from build123d import *

# Parameters (mm, degrees)
SKETCH_1_R          = 20
EXTRUDE_1_DEPTH     = 5
SKETCH_2_R          = 2
CUT_EXTRUDE_1_DEPTH = 29.722813233
SKETCH_3_R          = 3.5
CUT_EXTRUDE_2_DEPTH = 3
SKETCH_4_R          = 3
EXTRUDE_2_DEPTH     = 8
CUT_EXTRUDE_START   = -5
CUT_EXTRUDE_3_DEPTH = 5


with BuildPart() as part:
    # 草图1 → 凸台-拉伸1 (new body)
    with BuildSketch(Plane(origin=(0, 0, 0), x_dir=(1, 0, 0), z_dir=(0, 1, 0))):
        with Locations(Location((0, 0, 0), (0, 0, 270))):
            Circle(SKETCH_1_R)
    extrude(amount=EXTRUDE_1_DEPTH)

    # 草图2 → 切除-拉伸1 (cut, through all)
    with BuildSketch(Plane(origin=(0, 5, 0), x_dir=(1, 0, 0), z_dir=(0, 1, 0))):
        with Locations(Location((14, 0, 0), (0, 0, 270))):
            Circle(SKETCH_2_R)
        with Locations(Location((7, -12.124355653, 0), (0, 0, 270))):
            Circle(SKETCH_2_R)
        with Locations(Location((-7, -12.124355653, 0), (0, 0, 270))):
            Circle(SKETCH_2_R)
        with Locations(Location((-14, 0, 0), (0, 0, 270))):
            Circle(SKETCH_2_R)
        with Locations(Location((-7, 12.124355653, 0), (0, 0, 270))):
            Circle(SKETCH_2_R)
        with Locations(Location((7, 12.124355653, 0), (0, 0, 270))):
            Circle(SKETCH_2_R)
    extrude(amount=-CUT_EXTRUDE_1_DEPTH, mode=Mode.SUBTRACT)

    # 草图3 → 切除-拉伸2 (cut)
    with BuildSketch(Plane(origin=(0, 5, 0), x_dir=(1, 0, 0), z_dir=(0, 1, 0))):
        with Locations(Location((14, 0, 0), (0, 0, 270))):
            Circle(SKETCH_3_R)
        with Locations(Location((7, -12.124355653, 0), (0, 0, 270))):
            Circle(SKETCH_3_R)
        with Locations(Location((-7, -12.124355653, 0), (0, 0, 270))):
            Circle(SKETCH_3_R)
        with Locations(Location((-14, 0, 0), (0, 0, 270))):
            Circle(SKETCH_3_R)
        with Locations(Location((-7, 12.124355653, 0), (0, 0, 270))):
            Circle(SKETCH_3_R)
        with Locations(Location((7, 12.124355653, 0), (0, 0, 270))):
            Circle(SKETCH_3_R)
    extrude(amount=-CUT_EXTRUDE_2_DEPTH, mode=Mode.SUBTRACT)

    # 草图4 → 凸台-拉伸2 (add)
    with BuildSketch(Plane(origin=(0, 5, 0), x_dir=(1, 0, 0), z_dir=(0, 1, 0))):
        with Locations(Location((0, 0, 0), (0, 0, 270))):
            Circle(SKETCH_4_R)
    extrude(amount=EXTRUDE_2_DEPTH)

    # 草图5 → 切除-拉伸3 (cut)
    with BuildSketch(Plane(origin=(0, 13, 0), x_dir=(1, 0, 0), z_dir=(0, 1, 0)).offset(CUT_EXTRUDE_START)):
        with BuildLine():
            Line((2.014530219, -2.222986279), (1.985384834, 2.249054704))
            ThreePointArc((1.985384834, 2.249054704), (2.99993629, 0.019551319), (2.014530219, -2.222986279))
        make_face()
    extrude(amount=CUT_EXTRUDE_3_DEPTH, mode=Mode.SUBTRACT)


solid = part.part
Build history of the part. All positions in model axes, mm. A direction names the side the tool comes from. Coordinates: 2 decimals unless noted, no trailing zeros. Write each loop counter-clockwise with the first axis right and the second up, starting at its lowest first coordinate (ties: lowest second). Pieces come first, ordered by that corner, then holes. Notation, with made-up numbers: (44.5, 47) -> (92.5, 47) arc R26 ccw to (92.5, 69) -> close; hole circle Ø7 at (68, 47.25). An arc over 180 degrees is marked (long way). Use CSV: the item, a comma, the result in double quotes. Start each with the question number.
Q1. Cut at D-D, the plane x = 7. List the corners of the cut face in (y, z) (3 decimals).
Q2. Flat gauge pins, fed straight in: pin 1 Ø5.5 at (x, z) = (-7.5, 13.5) entering from +Y; pin 2 Ø2 at (x, z) = (12.5, 1) entering from +Y; pin 3 Ø6 at (y, z) = (4.5, -8.5) entering from -X. Where does each tip first touch, or does it go through?
Q3. Cut at B-B, the plane y = 3.5. List the corners of the cut face in (x, z).
Q4. Cut at A-A, the plane x = 13.5. List the corners of the cut face in (y, z).
Q5. Pull direction X, two halves, no side cores. Call faces 1 (the cylindrical face through (-2.93, 8.94, -0.65)), 2 (the flat face through (-9, 2, -11)), 3 (the cylindrical face through (-6.399, 1.014, 14.032)), 4 (the flat face through (0, 5, 4)): released by +X, released by -X, zero draft, split by the parting line, or undercut.
Q6. Cut at C-C, the plane z = 0. List the corners of the cut face in (x, y), then the cut area to 3 significant figures.
Q7. Drill centre lines: probe 1 along X at (y, z) = (1.4, 0); probe 2 along Z at (x, y) = (6.5, 4.5); probe 3 along Y at (x, z) = (-5.5, 13.5). Where is each one in solid material? Low to high.
Q8. 3-axis set-ups, long thin cutter, end or side, ignore diameter. For faces 5 (the flat face through (0, 13, 0)), 6 (the flat face through (-16, 2, 2)): which of +Z, -Z, +X, -X, +Y, -Y reach the whole face in a straight line?
Checked values:
1,outline,"(0, -18.735) -> (5, -18.735) -> (5, -15.624) -> (2, -15.624) -> (2, -14.124) -> (0, -14.124) -> close; (0, -10.124) -> (2, -10.124) -> (2, -8.624) -> (5, -8.624) -> (5, 8.624) -> (2, 8.624) -> (2, 10.124) -> (0, 10.124) -> close; (0, 14.124) -> (2, 14.124) -> (2, 15.624) -> (5, 15.624) -> (5, 18.735) -> (0, 18.735) -> close"
2,pin 1,"stops at y = 5"
2,pin 2,"stops at y = 2"
2,pin 3,"stops at x = -19.23"
3,outline,"circle Ø40 at (0, 0); hole circle Ø7 at (-14, 0); hole circle Ø7 at (-7, -12.12); hole circle Ø7 at (-7, 12.12); hole circle Ø7 at (7, -12.12); hole circle Ø7 at (7, 12.12); hole circle Ø7 at (14, 0)"
4,outline,"(0, -14.76) -> (5, -14.76) -> (5, -3.46) -> (2, -3.46) -> (2, -1.94) -> (0, -1.94) -> close; (0, 1.94) -> (2, 1.94) -> (2, 3.46) -> (5, 3.46) -> (5, 14.76) -> (0, 14.76) -> close"
5,face 1,"split by the parting line"
5,face 2,"undercut"
5,face 3,"undercut"
5,face 4,"zero draft"
6,outline,"(-20, 0) -> (-16, 0) -> (-16, 2) -> (-17.5, 2) -> (-17.5, 5) -> (-20, 5) -> close; (-12, 0) -> (12, 0) -> (12, 2) -> (10.5, 2) -> (10.5, 5) -> (3, 5) -> (3, 8) -> (2, 8) -> (2, 13) -> (-3, 13) -> (-3, 5) -> (-10.5, 5) -> (-10.5, 2) -> (-12, 2) -> close; (16, 0) -> (20, 0) -> (20, 5) -> (17.5, 5) -> (17.5, 2) -> (16, 2) -> close"
6,area,"185 mm²"
7,probe 1,"x = -20 to -16, -12 to 12, 16 to 20"
7,probe 2,"z = -18.91 to -15.59, -8.66 to 8.66, 15.59 to 18.91"
7,probe 3,"y = 0 to 2"
8,face 5,"+Z, -Z, +X, -X, +Y"
8,face 6,"+Y"
